Source: CAD feature listing. Evaluate the final solid. Frame: model axes, mm. Give positions to 0.01 mm unless a question says otherwise; leave off trailing zeros. Loops run counter-clockwise (first coordinate to the right, second up) from the corner with the lowest first, then second, coordinate; pieces in that order, holes last. Notation, with made-up numbers: (-27, 16.25) -> (22, 16.25) arc R25 ccw to (22, 30.25) -> close; hole circle Ø9 at (52.5, 3). An arc over 180 degrees is marked (long way). Put each result on its own line as item: value.
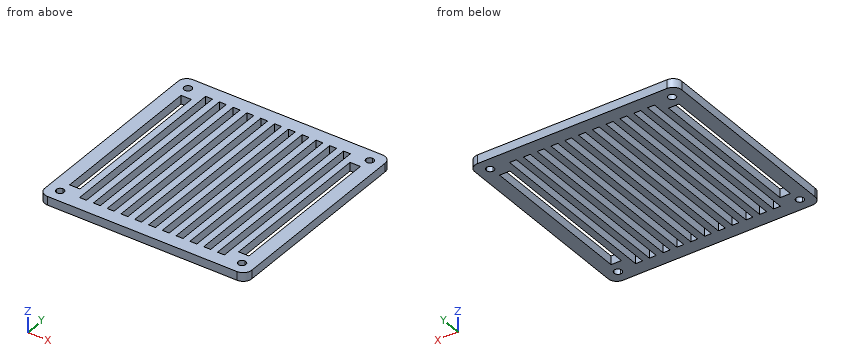
```python
from build123d import *

# Parameters (mm, degrees)
F0_W     = 120
F0_H     = 120
F1_DEPTH = 5
F2_R     = 5
F3_R     = 2.25
F4_DEPTH = 25
F5_W     = 6
F5_H     = 92
F6_DEPTH = 25
F7_DEPTH = 25
F8_DEPTH = 25


with BuildPart() as f1:
    # F0 (on Top) → F1 (new body)
    with BuildSketch(Plane.XY):
        with Locations((3.6000026762, 0.4973127641)):
            Rectangle(F0_W, F0_H)
    extrude(amount=F1_DEPTH)

    # F2
    f2_edges = [f1.edges().sort_by_distance(p)[0] for p in [
        (-56.399997, 60.497313, 2.5),
        (63.600003, 60.497313, 2.5),
        (63.600003, -59.502687, 2.5),
        (-56.399997, -59.502687, 2.5),
    ]]
    fillet(f2_edges, radius=F2_R)

    # F3 (on face) → F4 (cut)
    with BuildSketch(Plane.XY.offset(5)):
        with Locations((-49.1499973238, 53.2473127641)):
            Circle(F3_R)
        with BuildLine():
            ThreePointArc((56.3500026762, 50.9973127641), (57.9409929339, 51.6563225064), (58.6000026762, 53.2473127641))
            Line((58.6000026762, 53.2473127641), (56.3500026762, 53.2473127641))
            Line((56.3500026762, 53.2473127641), (56.3500026762, 50.9973127641))
        make_face()
        with BuildLine():
            Line((56.3500026762, 53.2473127641), (58.6000026762, 53.2473127641))
            ThreePointArc((58.6000026762, 53.2473127641), (57.9409929339, 54.8383030217), (56.3500026762, 55.4973127641))
            Line((56.3500026762, 55.4973127641), (56.3500026762, 53.2473127641))
        make_face()
        with BuildLine():
            Line((56.3500026762, 50.9973127641), (56.3500026762, 53.2473127641))
            Line((56.3500026762, 53.2473127641), (54.1000026762, 53.2473127641))
            ThreePointArc((54.1000026762, 53.2473127641), (54.7590124186, 51.6563225064), (56.3500026762, 50.9973127641))
        make_face()
        with BuildLine():
            Line((54.1000026762, 53.2473127641), (56.3500026762, 53.2473127641))
            Line((56.3500026762, 53.2473127641), (56.3500026762, 55.4973127641))
            ThreePointArc((56.3500026762, 55.4973127641), (54.7590124186, 54.8383030217), (54.1000026762, 53.2473127641))
        make_face()
        with BuildLine():
            ThreePointArc((-51.3999973238, -52.2526872359), (-50.7409875814, -53.8436774936), (-49.1499973238, -54.5026872359))
            Line((-49.1499973238, -54.5026872359), (-49.1499973238, -52.2526872359))
            Line((-49.1499973238, -52.2526872359), (-51.3999973238, -52.2526872359))
        make_face()
        with BuildLine():
            Line((-49.1499973238, -52.2526872359), (-49.1499973238, -54.5026872359))
            ThreePointArc((-49.1499973238, -54.5026872359), (-47.5590070661, -53.8436774936), (-46.8999973238, -52.2526872359))
            Line((-46.8999973238, -52.2526872359), (-49.1499973238, -52.2526872359))
        make_face()
        with BuildLine():
            Line((-51.3999973238, -52.2526872359), (-49.1499973238, -52.2526872359))
            Line((-49.1499973238, -52.2526872359), (-49.1499973238, -50.0026872359))
            ThreePointArc((-49.1499973238, -50.0026872359), (-50.7409875814, -50.6616969783), (-51.3999973238, -52.2526872359))
        make_face()
        with BuildLine():
            Line((-49.1499973238, -50.0026872359), (-49.1499973238, -52.2526872359))
            Line((-49.1499973238, -52.2526872359), (-46.8999973238, -52.2526872359))
            ThreePointArc((-46.8999973238, -52.2526872359), (-47.5590070661, -50.6616969783), (-49.1499973238, -50.0026872359))
        make_face()
        with BuildLine():
            ThreePointArc((54.1000026762, -52.2526872359), (54.7590124186, -53.8436774936), (56.3500026762, -54.5026872359))
            Line((56.3500026762, -54.5026872359), (56.3500026762, -52.2526872359))
            Line((56.3500026762, -52.2526872359), (54.1000026762, -52.2526872359))
        make_face()
        with BuildLine():
            Line((56.3500026762, -52.2526872359), (56.3500026762, -54.5026872359))
            ThreePointArc((56.3500026762, -54.5026872359), (57.9409929339, -53.8436774936), (58.6000026762, -52.2526872359))
            Line((58.6000026762, -52.2526872359), (56.3500026762, -52.2526872359))
        make_face()
        with BuildLine():
            Line((54.1000026762, -52.2526872359), (56.3500026762, -52.2526872359))
            Line((56.3500026762, -52.2526872359), (56.3500026762, -50.0026872359))
            ThreePointArc((56.3500026762, -50.0026872359), (54.7590124186, -50.6616969783), (54.1000026762, -52.2526872359))
        make_face()
        with BuildLine():
            Line((56.3500026762, -50.0026872359), (56.3500026762, -52.2526872359))
            Line((56.3500026762, -52.2526872359), (58.6000026762, -52.2526872359))
            ThreePointArc((58.6000026762, -52.2526872359), (57.9409929339, -50.6616969783), (56.3500026762, -50.0026872359))
        make_face()
    extrude(amount=-F4_DEPTH, mode=Mode.SUBTRACT)

    # F5 (on face) → F6 (cut)
    with BuildSketch(Plane.XY.offset(5)):
        with Locations((-45.3999973238, 0.4973127641)):
            Rectangle(F5_W, F5_H)
    extrude(amount=-F6_DEPTH, mode=Mode.SUBTRACT)

    # F5 (on face) → F7 (cut)
    with BuildSketch(Plane.XY.offset(5)):
        Polygon((-34.3999973238, 52.4973127641), (-38.3999973238, 52.4973127641), (-38.3999973238, 46.4973127641), (-38.3999973238, -45.5026872359), (-38.3999973238, -51.5026872359), (-34.3999973238, -51.5026872359), (-34.3999973238, -45.5026872359), (-34.3999973238, 46.4973127641), align=None)
        Polygon((-26.3999973238, 52.4973127641), (-30.3999973238, 52.4973127641), (-30.3999973238, 46.4973127641), (-30.3999973238, -45.5026872359), (-30.3999973238, -51.5026872359), (-26.3999973238, -51.5026872359), (-26.3999973238, -45.5026872359), (-26.3999973238, 46.4973127641), align=None)
        Polygon((-18.3999973238, 52.4973127641), (-22.3999973238, 52.4973127641), (-22.3999973238, 46.4973127641), (-22.3999973238, -45.5026872359), (-22.3999973238, -51.5026872359), (-18.3999973238, -51.5026872359), (-18.3999973238, -45.5026872359), (-18.3999973238, 46.4973127641), align=None)
        Polygon((-10.3999973238, 52.4973127641), (-14.3999973238, 52.4973127641), (-14.3999973238, 46.4973127641), (-14.3999973238, -45.5026872359), (-14.3999973238, -51.5026872359), (-10.3999973238, -51.5026872359), (-10.3999973238, -45.5026872359), (-10.3999973238, 46.4973127641), align=None)
        Polygon((-2.3999973238, 52.4973127641), (-6.3999973238, 52.4973127641), (-6.3999973238, 46.4973127641), (-6.3999973238, -45.5026872359), (-6.3999973238, -51.5026872359), (-2.3999973238, -51.5026872359), (-2.3999973238, -45.5026872359), (-2.3999973238, 46.4973127641), align=None)
        Polygon((5.6000026762, 52.4973127641), (1.6000026762, 52.4973127641), (1.6000026762, 46.4973127641), (1.6000026762, -45.5026872359), (1.6000026762, -51.5026872359), (5.6000026762, -51.5026872359), (5.6000026762, -45.5026872359), (5.6000026762, 46.4973127641), align=None)
        Polygon((13.6000026762, 46.4973127641), (13.6000026762, 52.4973127641), (9.6000026762, 52.4973127641), (9.6000026762, 46.4973127641), (9.6000026762, -45.5026872359), (9.6000026762, -51.5026872359), (13.6000026762, -51.5026872359), (13.6000026762, -45.5026872359), align=None)
        Polygon((21.6000026762, 46.4973127641), (21.6000026762, 52.4973127641), (17.6000026762, 52.4973127641), (17.6000026762, 46.4973127641), (17.6000026762, -45.5026872359), (17.6000026762, -51.5026872359), (21.6000026762, -51.5026872359), (21.6000026762, -45.5026872359), align=None)
        Polygon((29.6000026762, 46.4973127641), (29.6000026762, 52.4973127641), (25.6000026762, 52.4973127641), (25.6000026762, 46.4973127641), (25.6000026762, -45.5026872359), (25.6000026762, -51.5026872359), (29.6000026762, -51.5026872359), (29.6000026762, -45.5026872359), align=None)
        Polygon((37.6000026762, 46.4973127641), (37.6000026762, 52.4973127641), (33.6000026762, 52.4973127641), (33.6000026762, 46.4973127641), (33.6000026762, -45.5026872359), (33.6000026762, -51.5026872359), (37.6000026762, -51.5026872359), (37.6000026762, -45.5026872359), align=None)
        Polygon((45.6000026762, 46.4973127641), (45.6000026762, 52.4973127641), (41.6000026762, 52.4973127641), (41.6000026762, 46.4973127641), (41.6000026762, -45.5026872359), (41.6000026762, -51.5026872359), (45.6000026762, -51.5026872359), (45.6000026762, -45.5026872359), align=None)
    extrude(amount=-F7_DEPTH, mode=Mode.SUBTRACT)

    # F5 (on face) → F8 (cut)
    with BuildSketch(Plane.XY.offset(5)):
        with Locations((52.6000026762, 0.4973127641)):
            Rectangle(F5_W, F5_H)
    extrude(amount=-F8_DEPTH, mode=Mode.SUBTRACT)


solid = f1.part
```
(1) Section B-B on y = 44. Give the number of separate pieces and of enclosed holes in the cut face, then the cut area to 3 significant figures.
Calculated:
separate pieces: 14
enclosed holes: 0
area: 320 mm²
(2) Line query: probe 1 along Y at (x, z) = (43.5, 1.25); probe 2 along Y at (x, z) = (-49, 4.1); probe 3 along X at (y, z) = (54.5, 1.3). Output: solid intervals per line, ascending. Write a range as from..to.
Calculated:
probe 1: y = -59.5..-51.5, 52.5..60.5
probe 2: y = -59.5..-54.5, -50.01..51, 55.49..60.5
probe 3: x = -56.4..-51.02, -47.28..54.48, 58.22..63.6
(3) Section A-A on x = 27.5. Return loops of the section in (y, z), then the cut area to 3 significant figures.
Calculated:
outline: (-59.5, 0) -> (-51.5, 0) -> (-51.5, 5) -> (-59.5, 5) -> close; (52.5, 0) -> (60.5, 0) -> (60.5, 5) -> (52.5, 5) -> close
area: 80.0 mm²
